```python
from build123d import *

# Parameters (mm, degrees)
F0_R        = 9
F0_R_2      = 7.5
F0_R_3      = 6
F0_R_4      = 1.6
F0_R_5      = 2.5
F1_DEPTH    = 5
F2_T1_DEPTH = 5


# Not quite as in the source:
# - a fillet or chamfer that OpenCascade refuses, or shapes differently, is made with other operations: its cross-section is extruded or revolved along the edge and cut away or added


with BuildPart() as f1:
    # F0 (on Front) → F1 (new body)
    with BuildSketch(Plane.XZ):
        with BuildLine():
            Line((77.14561722, 20), (-0.2484538774, 20))
            Line((-0.2484538774, 20), (-29.0604767571, 20))
            Line((-29.0604767571, 20), (-31.3025846086, 20))
            Line((-31.3025846086, 20), (-31.3025846086, 0))
            Line((-31.3025846086, 0), (0, 0))
            Line((0, 0), (33.9829302539, 0))
            ThreePointArc((33.9829302539, 0), (34.7117105365, -4.7760782671), (31.6838696315, -8.540945299))
            Line((31.6838696315, -8.540945299), (0, -25))
            Line((0, -25), (0, -35))
            Line((0, -35), (120, -35))
            Line((120, -35), (90.9631787703, 12.2713973983))
            ThreePointArc((90.9631787703, 12.2713973983), (85.0616816679, 17.9365681271), (77.14561722, 20))
        make_face()
        with Locations((47.4024499138, -23)):
            Circle(F0_R, mode=Mode.SUBTRACT)
        with Locations((69.4024499138, -23)):
            Circle(F0_R_2, mode=Mode.SUBTRACT)
        with Locations((87.4024499138, -23)):
            Circle(F0_R_3, mode=Mode.SUBTRACT)
        with Locations((-20.1252056134, 10)):
            Circle(F0_R_4, mode=Mode.SUBTRACT)
        with Locations((69.8747943866, 10)):
            Circle(F0_R_5, mode=Mode.SUBTRACT)
    extrude(amount=F1_DEPTH)

    # F2: fillet of radius 5 on 2 edges, made by hand

    # F2_s2 → F2_t1 (join)
    with BuildSketch(Plane.XZ):
        with BuildLine():
            ThreePointArc((29.9588910165, -9.4370327313), (32.5111722793, -3.8136534352), (27.6539527219, 0))
            Line((27.6539527219, 0), (27.6539527219, 0.5))
            Line((27.6539527219, 0.5), (33.9829302539, 0.5))
            Line((33.9829302539, 0.5), (34.4050124686, 0.2680421685))
            ThreePointArc((34.4050124686, 0.2680421685), (31.914363461, -8.9846485721), (30.189384846, -9.8807360044))
            Line((30.189384846, -9.8807360044), (29.9588910165, -9.4370327313))
        make_face()
    extrude(amount=F2_T1_DEPTH)


solid = f1.part
```
Geometry check sheet. Reference: the model listing, model coordinates, mm. A direction names the side the tool comes from. Coordinates: 2 decimals unless noted, no trailing zeros. Loops run counter-clockwise (first coordinate to the right, second up) from the corner with the lowest first, then second, coordinate; pieces in that order, holes last. Notation, with made-up numbers: (-32, -16) - (-28, -16) arc R10 cw to (-28, -1) - close; hole circle Ø3 at (82.5, 74). An arc over 180 degrees is marked (long way). One line per item, written item: value. Start each with the question number.
(1) Tool access check on faces 1 (the flat face through (0, -2, -30)), 2 (the flat face through (-2, -2, 0)), 3 (the cylindrical face through (38.41, -2.46, -22.6)). Record the directions out of +Z, -Z, +X, -X, +Y, -Y that give a thin tool (end or side, any length) a straight path to the whole face; none if there is none.
(2) Mould release check, pull along Z, two halves, no side actions. Record for faces 4 (the flat face through (24, -2, 20)), 5 (the flat face through (15.19, -2.46, -17.11)), 6 (the flat face through (45, 0, -7)): released by +Z, released by -Z, zero draft, split by the parting line, or undercut.
(3) Cross-section at A-A on y = -4.2. Enter the section's corners in (x, z).
(4) Cross-section at D-D on x = -8.5. Enter the section's corners in (y, z), plus the area to 3 significant figures.
(5) Depth check by flat-ended pin: P1, Ø3, axis at y = -4, z = -17, coming from the -X side; P2, Ø2.5, axis at y = -2, z = -31.5, coming from the -X side. Enter the tip coordinate at first touch or a pass-through.
(6) Cross-section at B-B on z = 10. Enter the section's corners in (x, y).
(7) Cross-section at C-C on z = -23. Enter the section's corners in (x, y).
(8) Material ranges on line 1 (Z direction, x = 70, y = -3.65); line 2 (X direction, y = -2.85, z = -25.5); line 3 (X direction, y = -2.8, z = -17.5), recorded low to high. Write a range as [from, to].
Results below:
1. face 1: -Z, -X, +Y, -Y
1. face 2: -X, +Y, -Y
1. face 3: +Y, -Y
2. face 4: released by +Z
2. face 5: undercut
2. face 6: zero draft
3. outline: (-31.3, 0) - (27.65, 0) arc R5 cw to (29.96, -9.44) - (0, -25) - (0, -35) - (120, -35) - (90.96, 12.27) arc R16.22 ccw to (77.15, 20) - (-31.3, 20) - close; hole circle Ø3.2 at (-20.13, 10); hole circle Ø18 at (47.4, -23); hole circle Ø15 at (69.4, -23); hole circle Ø5 at (69.87, 10); hole circle Ø12 at (87.4, -23)
4. outline: (-5, 0) - (0, 0) - (0, 20) - (-5, 20) - close
4. area: 100 mm2
5. P1: stops at x = 12.51
5. P2: stops at x = 0
6. outline: (-31.3, -5) - (-21.73, -5) - (-21.73, 0) - (-31.3, 0) - close; (-18.53, -5) - (67.37, -5) - (67.37, 0) - (-18.53, 0) - close; (72.37, -5) - (92.36, -5) - (92.36, 0) - (72.37, 0) - close
7. outline: (3.85, -5) - (38.4, -5) - (38.4, 0) - (3.85, 0) - close; (56.4, -5) - (61.9, -5) - (61.9, 0) - (56.4, 0) - close; (76.9, -5) - (81.4, -5) - (81.4, 0) - (76.9, 0) - close; (93.4, -5) - (112.63, -5) - (112.63, 0) - (93.4, 0) - close
8. line 1: z = [-35, -30.48], [-15.52, 7.5], [12.5, 20]
8. line 2: x = [0, 38.76], [56.05, 62.33], [76.47, 81.95], [92.86, 114.16]
8. line 3: x = [14.44, 40.28], [54.53, 64.3], [74.5, 85], [89.8, 109.25]
